Geometry check sheet. Reference: the model listing, model coordinates, mm. Give positions to 0.01 mm unless a question says otherwise; leave off trailing zeros. Loops run counter-clockwise (first coordinate to the right, second up) from the corner with the lowest first, then second, coordinate; pieces in that order, holes last.
1. Material ranges on L1, parallel to X at y = 0.5, z = -142.5; L2, parallel to X at y = 7.5, z = 21; L3, parallel to X at y = 6, z = 95, recorded low to high.
2. Go/stop test with a flat-tipped pin: pin 1 Ø3 at (x, z) = (0, 140) entering from +Y. Record where the tip stops, or that it passes through.
3. Cross-section at A-A, the plane z = -8. Record the cut outline in (x, y), plus the area to 3 significant figures.
from build123d import *

# Parameters (mm, degrees)
BOSS_EXTRUDE1_DEPTH  = 224
SKETCH2_R            = 1.9
CUT_EXTRUDE1_DEPTH   = 449.194436663
SKETCH3_R            = 2.5
CUT_EXTRUDE2_DEPTH   = 225.445984593
M4_CLEARANCE_HOLE1_D = 4.8
CUT_EXTRUDE3_REACH   = 226.446
SKETCH6_R            = 5


with BuildPart() as part:
    # Sketch1 → Boss-Extrude1 (new, symmetric)
    with BuildSketch(Plane.XY):
        Polygon((0, 0), (0, -1.382978723), (10, -1.382978723), (10, 8.617021277), (3.448211747, 8.617021277), (3, 8.117021277), (3, 6.617021277), (7.587018089, 6.617021277), (7.587018089, 5.117021277), (3, 0), align=None)
    boss_extrude1 = extrude(amount=BOSS_EXTRUDE1_DEPTH, both=True)

    # Mirror1: Boss-Extrude1 across plane
    add(boss_extrude1.mirror(Plane(origin=(0, 0, 0), x_dir=(0, 0, 1), z_dir=(1, 0, 0))))

    # Sketch2 → Cut-Extrude1 (cut, through all)
    with BuildSketch(Plane.XY.offset(224)):
        with Locations((7.646716257, 0.97030502)):
            Circle(SKETCH2_R)
    cut_extrude1 = extrude(amount=-CUT_EXTRUDE1_DEPTH, mode=Mode.SUBTRACT)

    # Mirror2: Cut-Extrude1 across plane
    add(cut_extrude1.mirror(Plane(origin=(0, 0, 0), x_dir=(0, 0, 1), z_dir=(1, 0, 0))), mode=Mode.SUBTRACT)

    # Sketch3 → Cut-Extrude2 (cut, through all)
    with BuildSketch(Plane.XZ.offset(1.382978723)):
        with Locations(Location((0, 140, 0), (0, 0, 270))):
            Circle(SKETCH3_R)
        with Locations(Location((0, -140, 0), (0, 0, 270))):
            Circle(SKETCH3_R)
    extrude(amount=-CUT_EXTRUDE2_DEPTH, mode=Mode.SUBTRACT)

    # M4 Clearance Hole1 (through all)
    with Locations(Plane(origin=(0, -1.382978723, 0), x_dir=(-1, 0, 0), z_dir=(0, -1, 0))):
        with Locations((0, -214), (0, -194)):
            m4_clearance_hole1 = Hole(M4_CLEARANCE_HOLE1_D / 2)

    # Mirror3: M4 Clearance Hole1 across plane
    add(m4_clearance_hole1.mirror(Plane.XY), mode=Mode.SUBTRACT)

    # Cut-Extrude3: up to this face of the body (flat: up to its plane)
    cut_extrude3_end = Plane(part.part.faces().sort_by_distance((0, 0, 0))[0])
    # Sketch6 → Cut-Extrude3 (cut, up to the picked face)
    with BuildSketch(Plane(origin=(0, 8.617021277, 0), x_dir=(1, 0, 0), z_dir=(0, 1, 0)), mode=Mode.PRIVATE) as cut_extrude3_sk1:
        with Locations((0, -214)):
            Circle(SKETCH6_R)
    cut_extrude3_tool1 = split(extrude(cut_extrude3_sk1.sketch, amount=-CUT_EXTRUDE3_REACH, mode=Mode.PRIVATE), bisect_by=cut_extrude3_end, keep=Keep.BOTH, mode=Mode.PRIVATE)
    # Sketch6 → Cut-Extrude3 (cut, up to the picked face)
    with BuildSketch(Plane(origin=(0, 8.617021277, 0), x_dir=(1, 0, 0), z_dir=(0, 1, 0)), mode=Mode.PRIVATE) as cut_extrude3_sk2:
        with Locations((0, -194)):
            Circle(SKETCH6_R)
    cut_extrude3_tool2 = split(extrude(cut_extrude3_sk2.sketch, amount=-CUT_EXTRUDE3_REACH, mode=Mode.PRIVATE), bisect_by=cut_extrude3_end, keep=Keep.BOTH, mode=Mode.PRIVATE)
    cut_extrude3_1 = cut_extrude3_tool1.solids().sort_by(Axis((0, 8.617021, 214), (0, -1, 0)))[0]
    add(cut_extrude3_1, mode=Mode.SUBTRACT)
    cut_extrude3_2 = cut_extrude3_tool2.solids().sort_by(Axis((0, 8.617021, 194), (0, -1, 0)))[0]
    add(cut_extrude3_2, mode=Mode.SUBTRACT)
    cut_extrude3 = cut_extrude3_1 + cut_extrude3_2  # Cut-Extrude3 as one shape, for the pattern or mirror that repeats it

    # Mirror4: Cut-Extrude3 across plane
    add(cut_extrude3.mirror(Plane.XY), mode=Mode.SUBTRACT)


solid = part.part
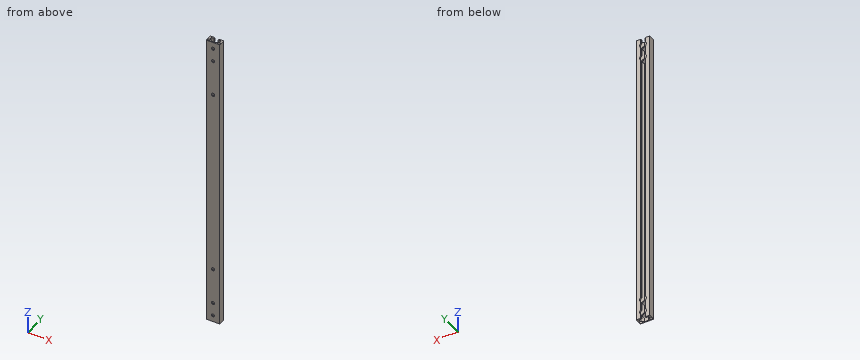
Result:
1. L1: x = -10 to -9.49, -5.81 to -3.45, 3.45 to 5.81, 9.49 to 10
1. L2: x = -10 to -3, 3 to 10
1. L3: x = -10 to -7.59, 7.59 to 10
2. pin 1: passes through
3. outline: (-10, -1.38) - (10, -1.38) - (10, 8.62) - (3.45, 8.62) - (3, 8.12) - (3, 6.62) - (7.59, 6.62) - (7.59, 5.12) - (3, 0) - (-3, 0) - (-7.59, 5.12) - (-7.59, 6.62) - (-3, 6.62) - (-3, 8.12) - (-3.45, 8.62) - (-10, 8.62) - close; hole circle Ø3.8 at (-7.65, 0.97); hole circle Ø3.8 at (7.65, 0.97)
3. area: 88.2 mm2
